Autodesk Inventor part; units mm, degrees
ref_plane "YZ Plane" through (0, 0, 0) normal (1, 0, 0) x (0, 1, 0)
ref_plane "XZ Plane" through (0, 0, 0) normal (0, 1, 0) x (-1, 0, 0)
ref_plane "XY Plane" through (0, 0, 0) normal (0, 0, 1) x (1, 0, 0)
sketch "Skizze1" plane through (0, 0, 0) normal (0, 1, 0) x (-1, 0, 0)
  line L0 (0, 0) -> (2, 0)
  line L1 (2, 0) -> (2, -14)
  line L2 (2, -14) -> (3, -14)
  line L3 (3, -14) -> (3, -82)
  line L4 (3, -82) -> (2, -82)
  line L5 (2, -82) -> (2, -96)
  line L6 (2, -96) -> (0, -96)
  line L7 (0, -96) -> (0, 0)
  point P0 (1, -96)
  dimension "d0" = 96
  dimension "d1" = 68
  dimension "d2" = 14
  dimension "d3" = 4
  dimension "d4" = 6
revolve "Umdrehung1" add sketch "Skizze1" angle 360 about axis through (0, 0, -96) along (0, 0, 1)
thread "Gewinde1"
thread "Gewinde2"
properties part number "1018"
Model file for the job. Use its own axes, mm. A direction names the side the tool comes from. Round coordinates to 2 decimals unless told otherwise and drop trailing zeros. Write each loop counter-clockwise with the first axis right and the second up, starting at its lowest first coordinate (ties: lowest second). Pieces come first, ordered by that corner, then holes. Notation, with made-up numbers: M -39.75,-25 L -10.75,-25 A16 cw -10.75,-14 Z; hole C 86.25,27 d9. An arc over 180 degrees is marked long. Put each result on its own line as item: value.
Item 1: Tool access for faces 1 (the flat face through (0, 0, -96)), 2 (the cylindrical face through (0, -2, -89)), 3 (the cylindrical face through (0, -2, -7)): list every direction of +Z, -Z, +X, -X, +Y, -Y with a clear straight run to the whole face (end or side of a thin tool).
Responses:
face 1: -Z, +X, -X, +Y, -Y
face 2: -Z
face 3: +Z
Item 2: Probe L1, parallel to Z at x = 2.15, y = -1.8; L2, parallel to Y at x = 0.1, z = -78.5; L3, parallel to X at y = 0.2, z = -63.5. List the from-to ranges inside material, lowest first. Write a range as from..to.
Responses:
L1: -82..-14
L2: -3..3
L3: -2.99..2.99
Item 3: Cut at D-D (z = -12.5). List the corners of the cut face in (x, y), and give its area (3 significant figures).
Responses:
outline: C 0,0 d4
area: 12.6 mm²
Item 4: Cut at C-C (z = -32.5). List the corners of the cut face in (x, y).
Responses:
outline: C 0,0 d6
Item 5: Cut at A-A (y = 0). List the corners of the cut face in (x, z).
Responses:
outline: M -3,-82 L -2,-82 L -2,-96 L 2,-96 L 2,-82 L 3,-82 L 3,-14 L 2,-14 L 2,0 L -2,0 L -2,-14 L -3,-14 Z
Item 6: Flat gauge pins, fed straight in: P1, Ø1, axis at y = -1, z = -40, coming from the -X side; P2, Ø1.5, axis at x = 2, y = -2.5, coming from the +Z side. Where does each tip first touch, or does it go through?
Responses:
P1: x = -2.96
P2: z = -14
